Verification items for this drawing (mm, ordinates from the low corner). Give positions to 0.01 mm unless a question says otherwise; leave off trailing zeros. Loops run counter-clockwise (first coordinate to the right, second up) from the corner with the lowest first, then second, coordinate; pieces in that order, holes last. Notation, with made-up numbers: M 86,-12.75 L 122,-12.75 A7 cw 122,-7.75 Z; hole C 43,1 d11. An arc over 180 degrees is marked long. Use one line per item in the form item = value.
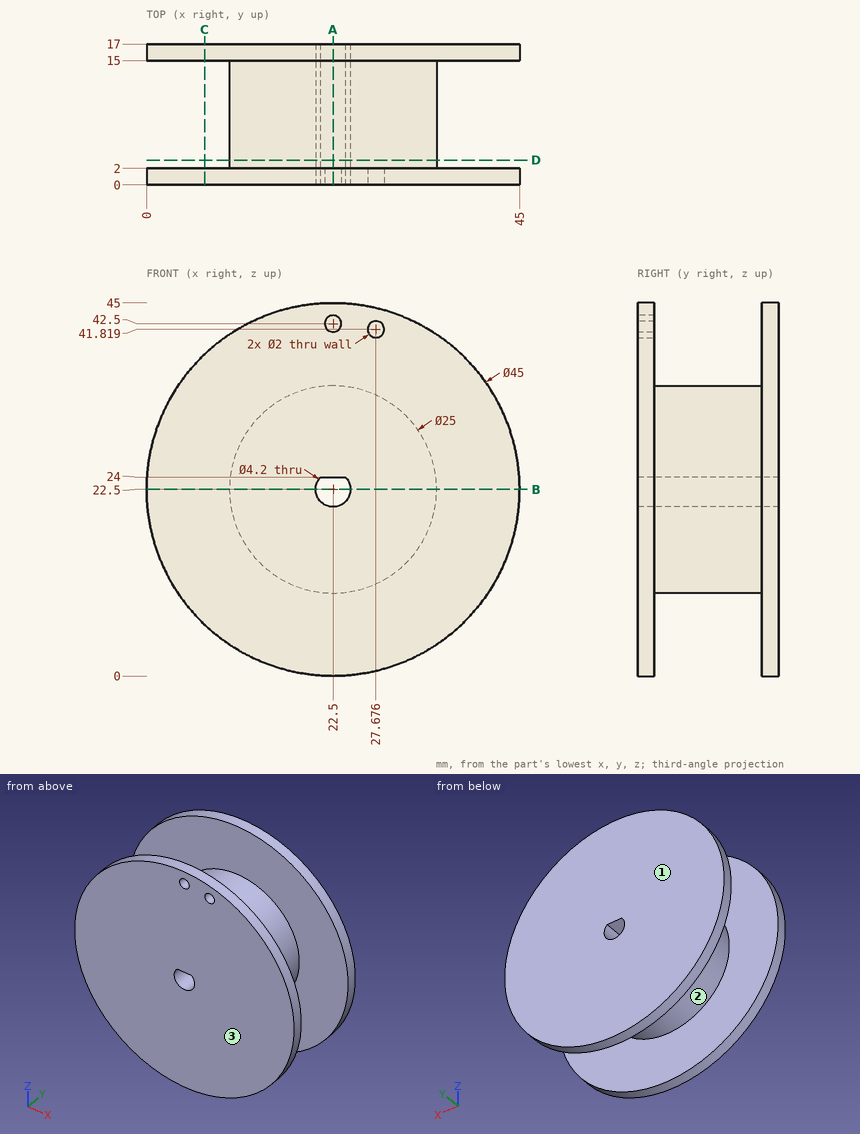
1) Section check A-A (x = 22.5). Record the cut outline in (y, z).
Evaluation:
outline = M 0,0 L 2,0 L 2,10 L 15,10 L 15,0 L 17,0 L 17,20.4 L 0,20.4 Z; M 0,24 L 17,24 L 17,45 L 15,45 L 15,35 L 2,35 L 2,41.5 L 0,41.5 Z; M 0,43.5 L 2,43.5 L 2,45 L 0,45 Z
2) Depth check by flat-ended pin: pin 1 Ø13.5 at (x, z) = (16.5, 14) entering from -Y; pin 2 Ø1.5 at (x, y) = (32, 2) entering from -Z; pin 3 Ø4 at (y, z) = (7.5, 34.5) entering from +X; pin 4 Ø4 at (y, z) = (9.5, 21) entering from +X. Enter the tip coordinate at first touch or a pass-through.
Evaluation:
pin_1 = 0
pin_2 = 1.77
pin_3 = 30
pin_4 = 35
3) Scan lines: line 1 (Y direction, x = 15, z = 38); line 2 (X direction, y = 9, z = 22.5); line 3 (Z direction, x = 22.5, y = 12.25). Record each from-to range of solid material in increasing order.
Evaluation:
line_1 = 0 to 2, 15 to 17
line_2 = 10 to 20.4, 24.6 to 35
line_3 = 10 to 20.4, 24 to 35
4) Section check C-C (x = 7). Record the cut outline in (y, z).
Evaluation:
outline = M 0,6.19 L 2,6.19 L 2,38.81 L 0,38.81 Z; M 15,6.19 L 17,6.19 L 17,38.81 L 15,38.81 Z
5) Section check D-D (y = 3). Record the cut outline in (x, z).
Evaluation:
outline = C 22.5,22.5 d25; hole M 21.03,24 A2.1 ccw long 23.97,24 Z
6) Section check B-B (z = 22.5). Record the cut outline in (x, y).
Evaluation:
outline = M 0,0 L 20.4,0 L 20.4,17 L 0,17 L 0,15 L 10,15 L 10,2 L 0,2 Z; M 24.6,0 L 45,0 L 45,2 L 35,2 L 35,15 L 45,15 L 45,17 L 24.6,17 Z
7) Release check for a two-part mould opening along Y. For the marked faces 1, 2 and 3 record: pulls with the +Y half, pulls with the -Y half, needs draft (parallel to the pull), parting line crosses it, or undercut.
Evaluation:
face_1 = pulls with the +Y half
face_2 = undercut
face_3 = pulls with the -Y half
